Input: part model. Units: mm. Frame: model coordinates. A direction names the side the tool comes from. Give positions to 0.01 mm unless a question says otherwise; leave off trailing zeros. Write each loop counter-clockwise with the first axis right and the second up, starting at its lowest first coordinate (ties: lowest second). Pieces come first, ordered by that corner, then holes.
Autodesk Inventor part; units mm, degrees
ref_plane "Work Plane5" through (-5.08, 0, -15.875) normal (0, 0, 1) x (1, 0, 0)
ref_plane "Work Plane6" through (-2.54, 0, -31.75) normal (-1, 0, 0) x (0, 0, 1)
ref_plane "YZ Plane" through (0, 0, 0) normal (1, 0, 0) x (0, 1, 0)
sketch "Sketch1" plane through (0, 0, 0) normal (0, 1, 0) x (-1, 0, 0)
  line L0 (0, 0) -> (5.08, 0)
  line L1 (5.08, 0) -> (5.08, -31.75)
  line L2 (5.08, -31.75) -> (0, -31.75)
  line L3 (0, -31.75) -> (0, 0)
  dimension "d0" = 5.08
  dimension "d1" = 31.75
extrude "Extrusion1" add sketch "Sketch1" along normal blind 1.5875
sketch "Sketch6" plane through (0, 1.5875, 0) normal (0, 1, 0) x (1, 0, 0)
  line L0 (-5.08, 0) -> (0, 0)
  line L1 (0, 31.75) -> (-5.08, 31.75)
  line L2 (0, 0) -> (-1.27, 0)
  line L3 (-1.27, 0) -> (-1.27, 31.75)
  line L4 (-1.27, 31.75) -> (0, 31.75)
  line L5 (0, 31.75) -> (0, 0)
  line L6 (-5.08, 31.75) -> (-5.08, 0)
  line L7 (-5.08, 0) -> (-3.81, 0)
  line L8 (-3.81, 0) -> (-3.81, 31.75)
  line L9 (-3.81, 31.75) -> (-5.08, 31.75)
  line L10 (-5.08, 31.75) -> (-5.08, 0)
  dimension "d19" = 31.75
  dimension "d20" = 1.27
  dimension "d21" = 31.75
  dimension "d22" = 1.27
extrude "Extrusion7" add sketch "Sketch6" along normal blind 11.43 contours L6 L1 L8 L0 | L3 L1 L5 L0
sketch "Sketch7" plane through (0, 1.5875, 0) normal (0, 1, 0) x (1, 0, 0)
  line L0 (-3.81, 0) -> (-1.27, 0)
  line L1 (-3.81, 31.75) -> (-3.81, 0)
  line L2 (-1.27, 0) -> (-3.81, 0)
  line L3 (-3.81, 0) -> (-3.81, 1.27)
  line L4 (-3.81, 1.27) -> (-1.27, 1.27)
  line L5 (-1.27, 1.27) -> (-1.27, 0)
  point P0 (0, 0)
  dimension "d25" = 1.27
extrude "Extrusion8" add sketch "Sketch7" along normal blind 1.27
sketch "Sketch8" plane through (-1.27, 1.5875, -31.75) normal (-1, 0, 0) x (0, 0, 1)
  line L0 (0, 11.43) -> (31.75, 11.43)
  line L1 (0, 11.43) -> (31.75, 11.43)
  line L2 (31.75, 11.43) -> (31.75, 10.16)
  line L3 (31.75, 10.16) -> (0, 10.16)
  line L4 (0, 10.16) -> (0, 11.43)
  point P0 (31.75, -1.5875)
  dimension "d28" = 31.75
  dimension "d29" = 1.27
extrude "Extrusion9" add sketch "Sketch8" along normal blind 0.508
chamfer "Chamfer1" distance 1.27 angle 45 1 edges at (-1.778, 13.0175, -15.875)
sketch "Sketch9" plane through (-1.27, 1.5875, -31.75) normal (-1, 0, 0) x (0, 0, 1)
  line L0 (30.48, 1.27) -> (31.75, 1.27)
  line L1 (31.75, 1.27) -> (30.48, 1.27)
  line L2 (30.48, 1.27) -> (30.48, 10.16)
  line L3 (30.48, 10.16) -> (31.75, 10.16)
  line L4 (31.75, 10.16) -> (31.75, 1.27)
  point P0 (31.75, -1.5875)
  dimension "d35" = 1.27
  dimension "d36" = 8.89
extrude "Extrusion10" add sketch "Sketch9" along normal blind 0.254
ref_plane "Work Plane5" through (-5.08, 0, -15.875) normal (0, 0, 1) x (1, 0, 0)
ref_plane "Work Plane6" through (-2.54, 0, -31.75) normal (-1, 0, 0) x (0, 0, 1)
mirror "Mirror4" about plane through (-2.54, 0, -31.75) normal (-1, 0, 0) of "Extrusion9", "Chamfer1", "Extrusion10"
mirror "Mirror5" about plane through (-5.08, 0, -15.875) normal (0, 0, 1) of "Extrusion10", "Extrusion8"
sketch "Sketch10" plane through (-3.81, 1.5875, -1.27) normal (1, 0, 0) x (0, 0, -1)
  line L0 (30.48, 1.27) -> (29.21, 1.27)
  line L1 (29.21, 1.27) -> (29.21, 10.16)
  line L2 (29.21, 10.16) -> (30.48, 10.16)
  line L3 (30.48, 10.16) -> (30.48, 1.27)
  point P0 (-1.27, -1.5875)
  dimension "d39" = 1.27
  dimension "d40" = 8.89
extrude "Extrusion11" add sketch "Sketch10" along normal blind 0.254
equation "\"d21\" = d19"
equation "\"d22\" = d20"
properties part number "cord holder"
Q1. Section D-D, the plane x = -4.1. Return the cut outline in (y, z).
Q2. Section B-B, the plane x = -2.65. Return the cut outline in (y, z).
Q3. Material intervals for line 1 along Z through (x, y) = (-3.65, 11.5); line 2 along X through (y, z) = (8, -9); line 3 along X through (y, z) = (12.5, -27), sorted ascending.
Q4. Pin query (flat end, axial travel): pin 1 (2 mm diameter, centred on x = -3.5, y = 8, fed in from -Z); pin 2 (2 mm diameter, centred on x = -3, z = -19.5, fed in from +Y). Return the tip coordinate at first contact, or that it passes through.
Q5. Section A-A, the plane y = 6.75. Return the cut outline in (x, z).
Q6. Mould query, pull axis Y, two halves, no side actions, for faces 5 (the flat face through (-3.556, 7, -1)), 6 (the flat face through (-3, 0, -16)), 7 (the flat face through (0, 6, -16)). Classes: +Y half, -Y half, draft (parallel to the pull), parting line (faces both ways), or undercut.
Q7. Access query for faces 1 (the flat face through (-5.08, 6, -16)), 2 (the flat face through (-3, 2.858, -1)), 3 (the flat face through (-3, 1.588, -16)), 4 (the flat face through (-3.928, 12.374, -16.097)). Directions: +Z, -Z, +X, -X, +Y, -Y. A direction counts if a zero-diameter tool reaches every point of the face in a straight line with its end or side. Return the directions, or none.
Solutions:
1. outline: (0, -31.75) - (12.55, -31.75) - (12.55, 0) - (0, 0) - close
2. outline: (0, -31.75) - (2.86, -31.75) - (2.86, -30.48) - (1.59, -30.48) - (1.59, -1.27) - (2.86, -1.27) - (2.86, 0) - (0, 0) - close
3. line 1: z = -31.75 to -30.48, -1.27 to 0
3. line 2: x = -5.08 to -3.81, -1.27 to 0
3. line 3: x = -5.08 to -4.05, -1.03 to 0
4. pin 1: stops at z = -31.75
4. pin 2: stops at y = 12.45
5. outline: (-5.08, -31.75) - (-3.56, -31.75) - (-3.56, -30.48) - (-3.81, -30.48) - (-3.81, -1.27) - (-3.56, -1.27) - (-3.56, 0) - (-5.08, 0) - close; (-1.52, -31.75) - (0, -31.75) - (0, 0) - (-1.52, 0) - (-1.52, -1.27) - (-1.27, -1.27) - (-1.27, -30.48) - (-1.52, -30.48) - close
6. face 5: undercut
6. face 6: -Y half
6. face 7: draft
7. face 1: +Z, -Z, -X, +Y, -Y
7. face 2: +Z, -Z
7. face 3: none
7. face 4: +Z, -Z, +Y
